Can you work these out from the drawing? Everything is in mm from the part's minimum corner. A direction names the side the tool comes from. Give positions to 0.01 mm unless a question says otherwise; leave off trailing zeros. Write each loop counter-clockwise with the first axis right and the second up, starting at its lowest first coordinate (ties: lowest second). Pieces come first, ordered by that corner, then holes. Notation, with made-up numbers: (-3, -25.5) -> (13, -25.5) arc R12 ccw to (13, -3.5) -> close; hole circle Ø6 at (45, 46.25). An arc over 180 degrees is marked (long way). Return JSON: item names as keys, results as strings.
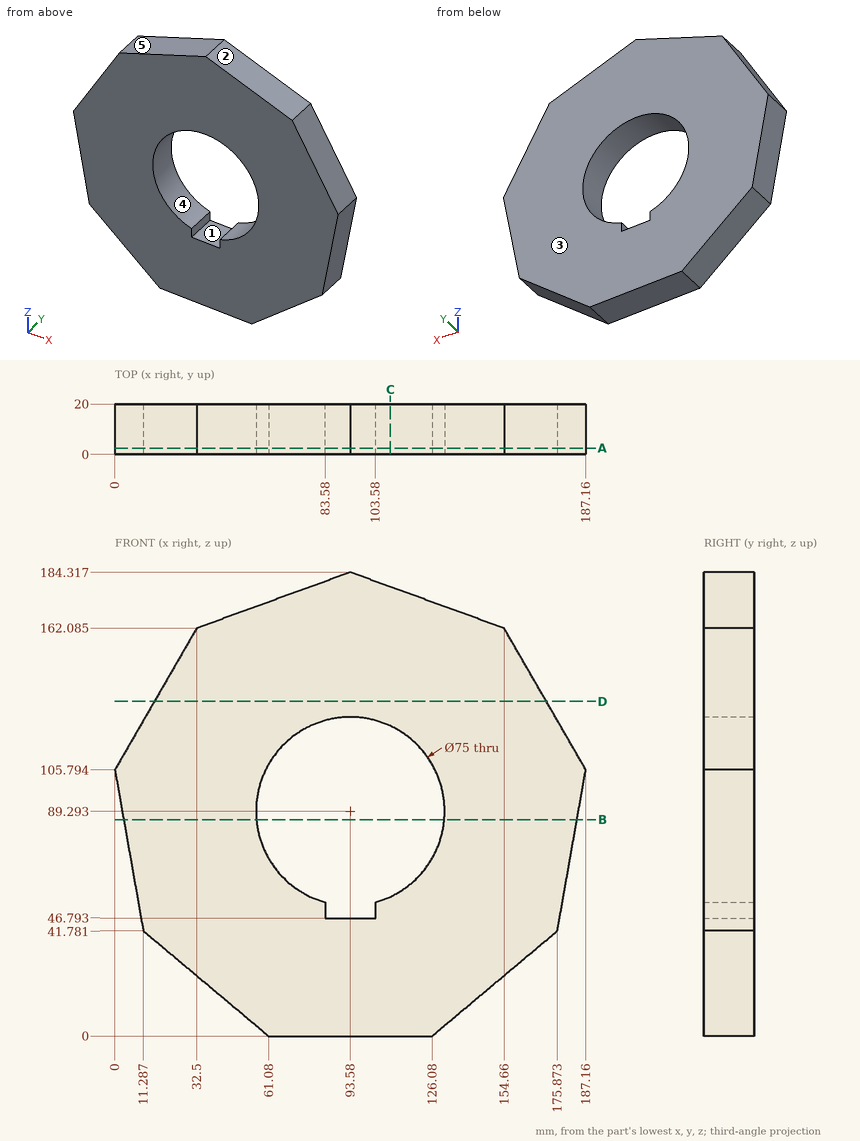
1. If I drill on line 1 (Z direction, x = 82, y = 1.25) (1 decimal); line 2 (X direction, y = 14, z = 117); line 3 (X direction, y = 14.75, z = 81), over which ranges is the centre line in solid material (lowest first)? Write a range as [from, to].
Taken from the geometry:
{"line 1": "z = [0, 53.6], [125, 180.1]", "line 2": "x = [6.47, 68.31], [118.85, 180.69]", "line 3": "x = [4.37, 57.01], [130.15, 182.79]"}
2. Suppose I cut it at B-B, the plane z = 86. List the corners of the cut face in (x, y) for me (1 decimal), and give its area (3 significant figures).
Taken from the geometry:
{"outline": "(3.5, 0) -> (56.2, 0) -> (56.2, 20) -> (3.5, 20) -> close; (130.9, 0) -> (183.7, 0) -> (183.7, 20) -> (130.9, 20) -> close", "area": "2,110 mm²"}
3. Suppose I cut it at C-C, the plane x = 109.5. List the corners of the cut face in (y, z) for me, and give its area (3 significant figures).
Taken from the geometry:
{"outline": "(0, 0) -> (20, 0) -> (20, 55.34) -> (0, 55.34) -> close; (0, 123.25) -> (20, 123.25) -> (20, 178.52) -> (0, 178.52) -> close", "area": "2,210 mm²"}
4. Which directions (+Z, -Z, +X, -X, +Y, -Y) give clear straight access to the entire face, cutting with the end or side of a thin tool? Please do the marked faces 1 and 2.
Taken from the geometry:
{"face 1": "+Y, -Y", "face 2": "+Z, +X, +Y, -Y"}
5. Suppose I cut it at A-A, the plane y = 2.5. List the corners of the cut face in (x, z) for me (1 decimal).
Taken from the geometry:
{"outline": "(0, 105.8) -> (11.3, 41.8) -> (61.1, 0) -> (126.1, 0) -> (175.9, 41.8) -> (187.2, 105.8) -> (154.7, 162.1) -> (93.6, 184.3) -> (32.5, 162.1) -> close; hole (83.6, 46.8) -> (103.6, 46.8) -> (103.6, 53.2) arc R37.5 ccw (long way) to (83.6, 53.2) -> close"}
6. Suppose I cut it at D-D, the plane z = 133. List the corners of the cut face in (x, y) for me, and give its area (4 significant figures).
Taken from the geometry:
{"outline": "(15.71, 0) -> (171.45, 0) -> (171.45, 20) -> (15.71, 20) -> close", "area": "3,115 mm²"}
7. For pin 1 Ø12 at (y, z) = (10.5, 121) entering from +X (1 decimal); pin 2 Ø4 at (y, z) = (15, 27.5) entering from -X; pin 3 Ø3 at (y, z) = (10, 49.5) entering from -X, each with a flat end and sliding along its axis, tell me the tip position at first contact or that it passes through.
Taken from the geometry:
{"pin 1": "stops at x = 181.8", "pin 2": "stops at x = 25.92", "pin 3": "stops at x = 9.66"}
8. If we mould it in two halves opening along Z, with no side actions, what happens to the marked faces 3, 4 and 5? For each: released by +Z, released by -Z, zero draft, split by the parting line, or undercut.
Taken from the geometry:
{"face 3": "zero draft", "face 4": "undercut", "face 5": "released by +Z"}
